```python
from build123d import *

# Parameters (mm, degrees)
EXTRUDE_1_DEPTH          = 15
CUT_EXTRUDE_1_DEPTH      = 25.839484697
CUT_EXTRUDE_1_DEPTH_BACK = 25.839484697
SKETCH_2_R               = 1.4
SKETCH_3_R               = 1.9
CUT_EXTRUDE_2_DEPTH      = 25.839484697
SKETCH_4_R               = 3
CUT_EXTRUDE_3_DEPTH      = 25.839484753


with BuildPart() as part:
    # 草图1 → 凸台-拉伸1 (new body)
    with BuildSketch(Plane(origin=(0, 0, 0), x_dir=(0, 0, -1), z_dir=(1, 0, 0))):
        Polygon((-14, 0), (0, 0), (0, 14), (-5, 14), (-14, 5), align=None)
    extrude(amount=EXTRUDE_1_DEPTH)

    # 草图2 → 切除-拉伸1 (cut, two sides: drawn at the far end of the back side and taken through both)
    with BuildSketch(Plane.XZ.offset(-CUT_EXTRUDE_1_DEPTH_BACK)):
        with Locations(Location((11.5, 6, 0), (0, 0, 225.584691403))):
            Circle(SKETCH_2_R)
        with Locations(Location((3.5, 6, 0), (0, 0, 225.584691403))):
            Circle(SKETCH_2_R)
    extrude(amount=CUT_EXTRUDE_1_DEPTH + CUT_EXTRUDE_1_DEPTH_BACK, mode=Mode.SUBTRACT)

    # 草图3 → 切除-拉伸2 (cut, through all)
    with BuildSketch(Plane(origin=(0, 0, 0), x_dir=(-1, 0, 0), z_dir=(0, 0, -1))):
        with Locations((-8.65, 7)):
            Circle(SKETCH_3_R)
    extrude(amount=-CUT_EXTRUDE_2_DEPTH, mode=Mode.SUBTRACT)

    # 草图4 → 切除-拉伸3 (cut, through all)
    with BuildSketch(Plane.XZ):
        with Locations((7.5, 14)):
            Circle(SKETCH_4_R)
    extrude(amount=-CUT_EXTRUDE_3_DEPTH, mode=Mode.SUBTRACT)


solid = part.part
```
For this review, take the finished solid that the model builds, in its own axes (mm). Round coordinates to 2 decimals unless told otherwise and drop trailing zeros. Write each loop counter-clockwise with the first axis right and the second up, starting at its lowest first coordinate (ties: lowest second). Pieces come first, ordered by that corner, then holes.
1) For line 1 along X through (y, z) = (9.5, 6); line 2 along Z through (x, y) = (3.5, 8); line 3 along Z through (x, y) = (3.5, 4.75), list the stretches that pass through material, from the lowest coordinate up.
Answer below:
line 1: x = 0 to 2.1, 4.9 to 10.1, 12.9 to 15
line 2: z = 0 to 4.6, 7.4 to 11
line 3: z = 0 to 4.6, 7.4 to 14
2) Take a section at C-C on y = 7. Give the boundary of the cut face in (x, z).
Answer below:
outline: (0, 0) - (6.75, 0) - (6.75, 11.1) arc R3 cw to (5.26, 12) - (0, 12) - close; (10.55, 0) - (15, 0) - (15, 12) - (10.55, 12) - (10.55, 7.03) arc R1.4 cw (long way) to (10.55, 4.97) - close; hole circle Ø2.8 at (3.5, 6)
3) Mouldability with a two-part tool opening along Z and no side actions: class faces 1 (the face through (11.816, 7.098, 4.636)), 2 (the face through (7, 5, 0)), 3 (the face through (15, 6, 6)) as +Z half, -Z half, draft (parallel to the pull), parting line (faces both ways), or undercut.
Answer below:
face 1: undercut
face 2: -Z half
face 3: draft
4) Take a section at D-D on z = 1.5. Give the boundary of the cut face in (x, y).
Answer below:
outline: (0, 0) - (15, 0) - (15, 14) - (0, 14) - close; hole circle Ø3.8 at (8.65, 7)
5) Take a section at B-B on z = 7. Give the boundary of the cut face in (x, y), then the cut area to 3 significant figures.
Answer below:
outline: (0, 0) - (2.52, 0) - (2.52, 12) - (0, 12) - close; (4.48, 0) - (10.52, 0) - (10.52, 6.66) arc R1.9 cw (long way) to (10.52, 7.34) - (10.52, 12) - (4.48, 12) - close; (12.48, 0) - (15, 0) - (15, 12) - (12.48, 12) - close
area: 122 mm2
6) Insertion check: pin 1 Ø1 at (x, z) = (10, 9.5) entering from +Y. The pin has a flat end and moves straight along its axis. Give the tip position at first contact, or say it passes through.
Answer below:
pin 1: stops at y = 10
7) Take a section at A-A on x = 4. Give the boundary of the cut face in (y, z).
Answer below:
outline: (0, 0) - (14, 0) - (14, 4.69) - (0, 4.69) - close; (0, 7.31) - (11.69, 7.31) - (5, 14) - (0, 14) - close
